from build123d import *

# Parameters (mm, degrees)
F0_R     = 63.5
F0_R_2   = 59.69
F1_DEPTH = 127
F2_W     = 127
F2_H     = 76.2
F2_W_2   = 116.3319997936
F2_H_2   = 65.5319997936
F3_DEPTH = 127
F4_R     = 12.7
F5_R     = 5.08
F6_R     = 5.08
F7_R     = 5.08
F8_R     = 5.08


with BuildPart() as f1:
    # F0 (on Top) → F1 (new body)
    with BuildSketch(Plane.XY):
        Circle(F0_R)
        Circle(F0_R_2, mode=Mode.SUBTRACT)
    extrude(amount=F1_DEPTH)

    # F2 (on Top) → F3 (join)
    with BuildSketch(Plane.XY):
        with Locations((63.5, -38.1)):
            Rectangle(F2_W, F2_H)
        with Locations((63.5, -38.1)):
            Rectangle(F2_W_2, F2_H_2, mode=Mode.SUBTRACT)
    extrude(amount=F3_DEPTH)

    # F4
    f4_edges = [f1.edges().sort_by_distance(p)[0] for p in [
        (0, -63.5, 63.5),
    ]]
    fillet(f4_edges, radius=F4_R)

    # F5
    f5_edges = [f1.edges().sort_by_distance(p)[0] for p in [
        (63.5, 0, 63.5),
    ]]
    fillet(f5_edges, radius=F5_R)

    # F6
    f6_edges = [f1.edges().sort_by_distance(p)[0] for p in [
        (127, 0, 63.5),
    ]]
    fillet(f6_edges, radius=F6_R)

    # F7
    f7_edges = [f1.edges().sort_by_distance(p)[0] for p in [
        (127, -76.2, 63.5),
    ]]
    fillet(f7_edges, radius=F7_R)

    # F8
    f8_edges = [f1.edges().sort_by_distance(p)[0] for p in [
        (0, -76.2, 63.5),
    ]]
    fillet(f8_edges, radius=F8_R)


solid = f1.part
Could you check a few things on this model? Use its own coordinates, in mm. A direction names the side the tool comes from. Give positions to 0.01 mm unless a question says otherwise; leave off trailing zeros. Order: outer loops, then holes, each group sorted by start corner. A loop starts at its lowest first (then second) coordinate and runs counter-clockwise, first axis right, second up. Notation, with made-up numbers: (-9, 88.25) - (29, 88.25) arc R8 cw to (29, 102.25) - close; hole circle Ø8 at (36.5, 10). An arc over 180 degrees is marked (long way). One line per question, with ' | ' between items. Start each with the question number.
Item 1: I want a section at C-C on x = 9.5. Write out the boundary of the cut face in (y, z).
Item 2: For faces 1 (the flat face through (0, -30, 63)), 2 (the cylindrical face through (64.9, 1.39, 64.39)), which set-ups out of +Z, -Z, +X, -X, +Y, -Y let a thin tool reach every point of the face, with its end or its side?
Item 3: Thinking about a two-plate mould opening in X: for faces 3 (the cylindrical face through (125.551, -74.672, 64.389)), 4 (the cylindrical face through (-40.79, 43.58, 62.61)), 5 (the flat face through (95, 0, 63)), which applies, pulls with the +X half, pulls with the -X half, needs draft (parallel to the pull), parting line crosses it, or undercut?
Item 4: I need wall thicknesses on probe 1 along X at (y, z) = (-15, 55); probe 2 along X at (y, z) = (-34, 14); probe 3 along X at (y, z) = (-5, 10). Which ranges of each line are inside material? Lowest first, please. Write a range as [from, to].
Item 5: I want a section at D-D on z = 107. Give the number of separate pieces and of enclosed holes in the cut face, then the cut area to 3 significant figures.
Item 6: I want a section at B-B on y = 47. Write out the boundary of the cut face in (x, z), then the cut area to 3 significant figures.
Item 7: I'm going to push flat-ended pins straight in: pin 1 Ø12 at (x, z) = (30, 82) entering from +Y; pin 2 Ø1 at (x, z) = (101, 52.5) entering from +Y; pin 3 Ø2 at (y, z) = (-42.5, 51.5) entering from -X. Where does each tip first touch, or does it pass through?
Item 8: I want a section at A-A on x = 95. Write out the boundary of the cut face in (y, z).
Verdict:
1) outline: (-76.2, 0) - (-70.87, 0) - (-70.87, 127) - (-76.2, 127) - close; (-62.79, 0) - (-58.93, 0) - (-58.93, 127) - (-62.79, 127) - close; (-5.33, 0) - (0, 0) - (0, 127) - (-5.33, 127) - close; (58.93, 0) - (62.79, 0) - (62.79, 127) - (58.93, 127) - close
2) face 1: +Z, -Z | face 2: +Z, -Z, +X, +Y
3) face 3: pulls with the +X half | face 4: undercut | face 5: needs draft
4) probe 1: [-61.7, -57.77], [0, 5.33], [57.77, 61.7], [121.67, 127] | probe 2: [-53.63, -49.06], [0, 5.33], [49.06, 53.63], [121.67, 127] | probe 3: [-63.3, -59.48], [0, 127]
5) separate pieces: 1 | enclosed holes: 3 | area: 3,500 mm^2
6) outline: (-42.7, 0) - (-36.8, 0) - (-36.8, 127) - (-42.7, 127) - close; (36.8, 0) - (42.7, 0) - (42.7, 127) - (36.8, 127) - close | area: 1,500 mm^2
7) pin 1: y = 58.79 | pin 2: y = 0 | pin 3: x = -48.06
8) outline: (-76.2, 0) - (-70.87, 0) - (-70.87, 127) - (-76.2, 127) - close; (-5.33, 0) - (0, 0) - (0, 127) - (-5.33, 127) - close
